Verification items for this drawing (mm, ordinates from the low corner). A direction names the side the tool comes from. Give positions to 0.01 mm unless a question says otherwise; leave off trailing zeros. Write each loop counter-clockwise with the first axis right and the second up, starting at its lowest first coordinate (ties: lowest second). Pieces come first, ordered by that corner, then holes. Notation, with made-up numbers: M -22,40.25 L 33,40.25 A34 cw 33,76.25 Z; hole C -24,-38 d5. An arc over 180 degrees is marked long. Write each question's results on one line, items separated by ' | '.
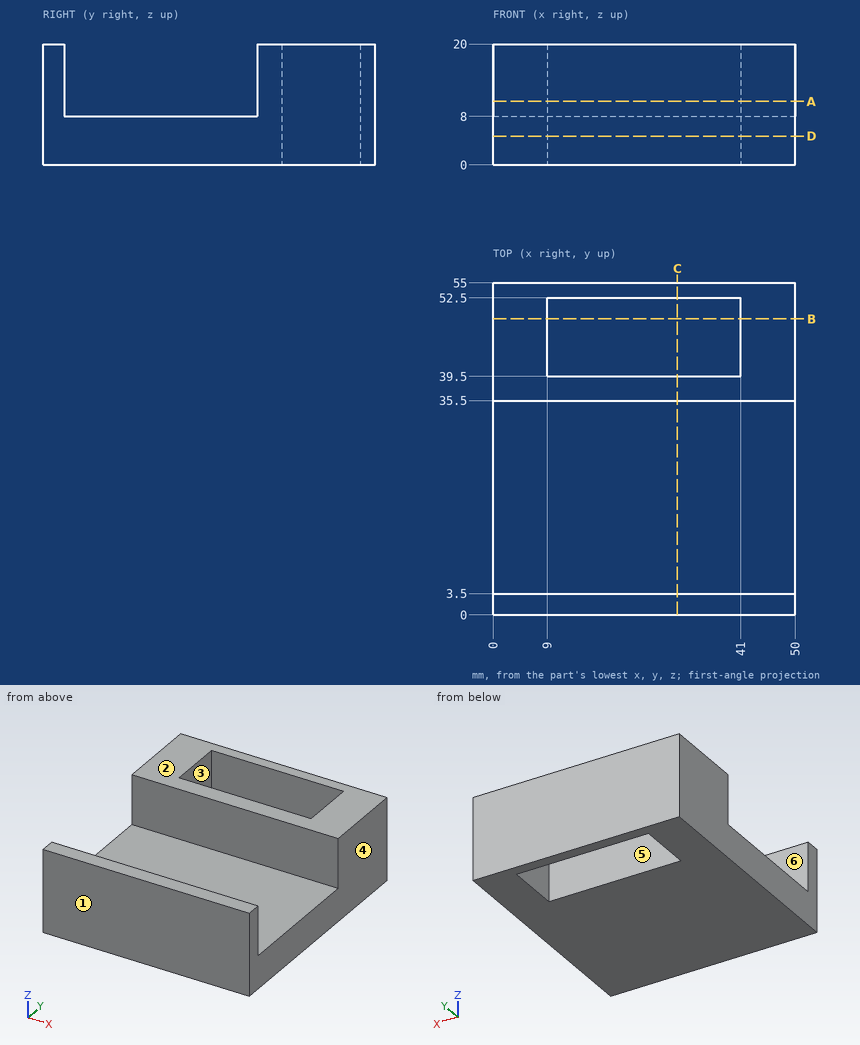
Q1. Section check B-B (y = 49). Enter the section's corners in (x, z).
Answer key:
outline: M 0,0 L 9,0 L 9,20 L 0,20 Z; M 41,0 L 50,0 L 50,20 L 41,20 Z
Q2. Material ranges on probe 1 along Y at (x, z) = (30.5, 9.5); probe 2 along Y at (x, z) = (46.5, 9); probe 3 along Y at (x, z) = (31, 3.75), recorded low to high. Write a range as [from, to].
Answer key:
probe 1: y = [0, 3.5], [35.5, 39.5], [52.5, 55] | probe 2: y = [0, 3.5], [35.5, 55] | probe 3: y = [0, 39.5], [52.5, 55]
Q3. Section check A-A (z = 10.5). Enter the section's corners in (x, y), then the cut area to 3 significant figures.
Answer key:
outline: M 0,0 L 50,0 L 50,3.5 L 0,3.5 Z; M 0,35.5 L 50,35.5 L 50,55 L 0,55 Z; hole M 9,39.5 L 41,39.5 L 41,52.5 L 9,52.5 Z | area: 734 mm2
Q4. Section check C-C (x = 30.5). Enter the section's corners in (y, z).
Answer key:
outline: M 0,0 L 39.5,0 L 39.5,20 L 35.5,20 L 35.5,8 L 3.5,8 L 3.5,20 L 0,20 Z; M 52.5,0 L 55,0 L 55,20 L 52.5,20 Z
Q5. Section check D-D (z = 4.75). Enter the section's corners in (x, y).
Answer key:
outline: M 0,0 L 50,0 L 50,55 L 0,55 Z; hole M 9,39.5 L 41,39.5 L 41,52.5 L 9,52.5 Z
Q6. Depth check by flat-ended pin: P1, Ø4, axis at x = 31.5, y = 29, coming from the +Z side. Enter the tip coordinate at first touch or a pass-through.
Answer key:
P1: stops at z = 8
Q7. Release check for a two-part mould opening along Y. For the marked faces 1, 2 and 3 record: released by +Y, released by -Y, zero draft, split by the parting line, or undercut.
Answer key:
face 1: released by -Y | face 2: zero draft | face 3: undercut
Q8. Access from +Z, -Z, +X, -X, +Y, -Y to the whole of each face (thin tool, end or side, straight path). Record for the marked faces 4, 5 and 6.
Answer key:
face 4: +Z, -Z, +X, +Y, -Y | face 5: +Z, -Z | face 6: +Z, +X, -X
